Can you work these out from the model? Positions are in its coordinate system, mm. Give positions to 0.01 mm unless a question says otherwise; leave off trailing zeros. Write each loop counter-clockwise with the first axis right and the second up, starting at its lowest first coordinate (ties: lowest second). Pieces come first, ordered by that corner, then holes.
1. Suppose I cut it at D-D (y = -104.5). Please give me the cut outline in (x, z) (3 decimals), and give its area (3 significant figures).
2. Suppose I cut it at A-A (x = 50.8). Please give me the cut outline in (y, z) (3 decimals).
3. If I drill on probe 1 along Y at (x, z) = (50.8, 1.45); probe 2 along X at (y, z) = (-73, 0.9); probe 3 along X at (y, z) = (49, 2.7), over which ranges is the centre line in solid material (lowest first)?
4. Suppose I cut it at C-C (x = -8.5). Please give me the cut outline in (y, z) (3 decimals), and give its area (3 significant figures).
5. Suppose I cut it at B-B (z = 0.5). Please give me the cut outline in (x, y) (3 decimals).
```python
from build123d import *

# Parameters (mm, degrees)
SKETCH1_W                  = 241.3
SKETCH1_H                  = 127
BOSS_EXTRUDE1_DEPTH        = 3.175
F_9_0_196_DIAMETER_HOLE1_D = 4.9784
CUT_EXTRUDE1_DEPTH         = 137.377245628


with BuildPart() as part:
    # Sketch1 → Boss-Extrude1 (new body)
    with BuildSketch(Plane(origin=(0, 0, 0), x_dir=(0, 1, 0), z_dir=(0, 0, 1))):
        Rectangle(SKETCH1_W, SKETCH1_H)
    extrude(amount=BOSS_EXTRUDE1_DEPTH)

    # #9 (0.196) Diameter Hole1 (through all)
    with Locations(Plane.XY.offset(3.175)):
        with Locations((50.8, 73.025), (50.8, -73.025), (50.8, -47.625), (50.8, 47.625)):
            Hole(F_9_0_196_DIAMETER_HOLE1_D / 2)

    # Sketch4 → Cut-Extrude1 (cut, through all)
    with BuildSketch(Plane.XY.offset(3.175)):
        with BuildLine():
            Line((-63.5, -44.45), (-63.5, -120.65))
            Line((-63.5, -120.65), (63.5, -120.65))
            ThreePointArc((63.5, -120.65), (-7.189698378, -94.53283063), (-63.5, -44.45))
        make_face()
    extrude(amount=-CUT_EXTRUDE1_DEPTH, mode=Mode.SUBTRACT)


solid = part.part
```
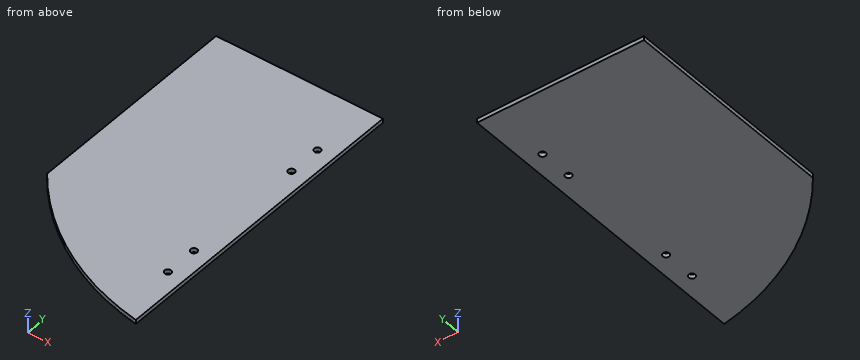
Checks:
1. outline: (11.583, 0) - (63.5, 0) - (63.5, 3.175) - (11.583, 3.175) - close
1. area: 165 mm2
2. outline: (-118.085, 0) - (-75.514, 0) - (-75.514, 3.175) - (-118.085, 3.175) - close; (-70.536, 0) - (-50.114, 0) - (-50.114, 3.175) - (-70.536, 3.175) - close; (-45.136, 0) - (45.136, 0) - (45.136, 3.175) - (-45.136, 3.175) - close; (50.114, 0) - (70.536, 0) - (70.536, 3.175) - (50.114, 3.175) - close; (75.514, 0) - (120.65, 0) - (120.65, 3.175) - (75.514, 3.175) - close
3. probe 1: y = -118.09 to -75.51, -70.54 to -50.11, -45.14 to 45.14, 50.11 to 70.54, 75.51 to 120.65
3. probe 2: x = -36.7 to 48.31, 53.29 to 63.5
3. probe 3: x = -63.5 to 48.73, 52.87 to 63.5
4. outline: (-93.74, 0) - (120.65, 0) - (120.65, 3.175) - (-93.74, 3.175) - close
4. area: 681 mm2
5. outline: (-63.5, -44.45) arc R203.2 ccw to (63.5, -120.65) - (63.5, 120.65) - (-63.5, 120.65) - close; hole circle Ø4.978 at (50.8, -73.025); hole circle Ø4.978 at (50.8, -47.625); hole circle Ø4.978 at (50.8, 47.625); hole circle Ø4.978 at (50.8, 73.025)
